```python
from build123d import *

# Parameters (mm, degrees)
F0_R     = 1.5875
F1_DEPTH = 1.5875
F2_R     = 0.79375
F5_DEPTH = 1.5885


with BuildPart() as f1:
    # F0 (on Top) → F1 (new body)
    with BuildSketch(Plane.XY):
        with BuildLine():
            Line((0, 52.563247), (0, 0))
            Line((0, 0), (98.425, 0))
            Line((98.425, 0), (98.425, 46.388994))
            Line((98.425, 46.388994), (14.2875, 46.388994))
            Line((14.2875, 46.388994), (14.2875, 98.425))
            Line((14.2875, 98.425), (31.75, 98.425))
            ThreePointArc((31.75, 98.425), (44.45, 111.125), (31.75, 123.825))
            Line((31.75, 123.825), (0, 123.825))
            Line((0, 123.825), (0, 92.250747))
            ThreePointArc((0, 92.250747), (2.80633, 91.088327), (3.96875, 88.281997))
            Line((3.96875, 88.281997), (3.96875, 56.531997))
            ThreePointArc((3.96875, 56.531997), (2.80633, 53.725667), (0, 52.563247))
        make_face()
        with BuildLine():
            Line((71.4375, 6.35), (39.6875, 6.35))
            ThreePointArc((39.6875, 6.35), (35.71875, 10.31875), (39.6875, 14.2875))
            Line((39.6875, 14.2875), (71.4375, 14.2875))
            ThreePointArc((71.4375, 14.2875), (75.40625, 10.31875), (71.4375, 6.35))
        make_face(mode=Mode.SUBTRACT)
        with BuildLine():
            Line((71.4375, 31.307744), (39.6875, 31.307744))
            ThreePointArc((39.6875, 31.307744), (35.71875, 35.276494), (39.6875, 39.245244))
            Line((39.6875, 39.245244), (71.4375, 39.245244))
            ThreePointArc((71.4375, 39.245244), (75.40625, 35.276494), (71.4375, 31.307744))
        make_face(mode=Mode.SUBTRACT)
        with Locations((31.75, 111.125)):
            Circle(F0_R, mode=Mode.SUBTRACT)
        with BuildLine():
            ThreePointArc((39.6875, 39.245244), (35.71875, 35.276494), (39.6875, 31.307744))
            Line((39.6875, 31.307744), (71.4375, 31.307744))
            ThreePointArc((71.4375, 31.307744), (75.40625, 35.276494), (71.4375, 39.245244))
            Line((71.4375, 39.245244), (39.6875, 39.245244))
        make_face()
        with BuildLine():
            ThreePointArc((39.6875, 14.2875), (35.71875, 10.31875), (39.6875, 6.35))
            Line((39.6875, 6.35), (71.4375, 6.35))
            ThreePointArc((71.4375, 6.35), (75.40625, 10.31875), (71.4375, 14.2875))
            Line((71.4375, 14.2875), (39.6875, 14.2875))
        make_face()
    extrude(amount=F1_DEPTH)

    # F2
    f2_edges = [f1.edges().sort_by_distance(p)[0] for p in [
        (14.2875, 98.425, 0.79375),
        (14.2875, 46.388994, 0.79375),
        (98.425, 46.388994, 0.79375),
        (98.425, 0, 0.79375),
    ]]
    fillet(f2_edges, radius=F2_R)

    # F3: F1 across plane


with BuildPart() as f1_1:
    add(f1.part)
    add(f1.part.mirror(Plane.YZ))

    # F4 (on face) → F5 (cut, through all)
    with BuildSketch(Plane.XY.offset(1.5875)):
        with BuildLine():
            ThreePointArc((-71.4375, 27.163247), (-75.40625, 23.194497), (-71.4375, 19.225747))
            Line((-71.4375, 19.225747), (-39.6875, 19.225747))
            ThreePointArc((-39.6875, 19.225747), (-35.71875, 23.194497), (-39.6875, 27.163247))
            Line((-39.6875, 27.163247), (-71.4375, 27.163247))
        make_face()
        with BuildLine():
            Line((71.4375, 39.245244), (39.6875, 39.245244))
            ThreePointArc((39.6875, 39.245244), (35.71875, 35.276494), (39.6875, 31.307744))
            Line((39.6875, 31.307744), (71.4375, 31.307744))
            ThreePointArc((71.4375, 31.307744), (75.40625, 35.276494), (71.4375, 39.245244))
        make_face()
        with BuildLine():
            ThreePointArc((39.6875, 14.2875), (35.71875, 10.31875), (39.6875, 6.35))
            Line((39.6875, 6.35), (71.4375, 6.35))
            ThreePointArc((71.4375, 6.35), (75.40625, 10.31875), (71.4375, 14.2875))
            Line((71.4375, 14.2875), (39.6875, 14.2875))
        make_face()
    extrude(amount=-F5_DEPTH, mode=Mode.SUBTRACT)


solid = f1_1.part
```
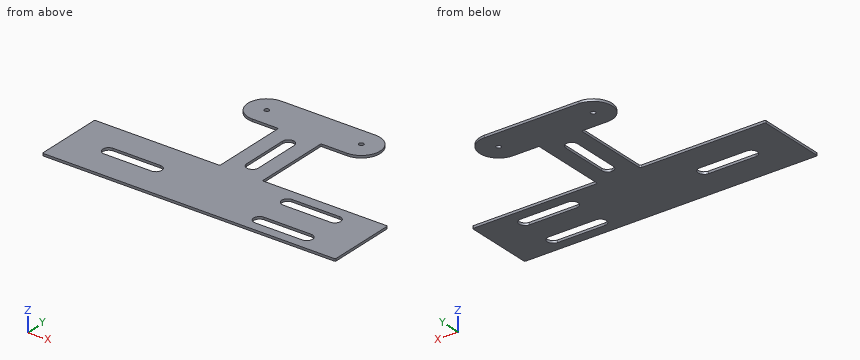
Model file for the job. Use its own axes, mm. Give positions to 0.01 mm unless a question says otherwise; leave off trailing zeros. Loops run counter-clockwise (first coordinate to the right, second up) from the corner with the lowest first, then second, coordinate; pieces in that order, holes last. Notation, with made-up numbers: (54.5, -28) -> (66.5, -28) arc R23 cw to (66.5, 4) -> close; hole circle Ø8 at (-27.5, 9.5). An arc over 180 degrees is marked (long way). Write each question's results on one line, items separated by ' | '.
(1) Cut at D-D on y = 95. List the corners of the cut face in (x, z).
Geometry results:
outline: (-14.29, 0) -> (14.29, 0) -> (14.29, 1.59) -> (-14.29, 1.59) -> close
(2) Cut at B-B on y = 24.5. List the corners of the cut face in (x, z) (1 decimal).
Geometry results:
outline: (-98.4, 0) -> (-75.2, 0) -> (-75.2, 1.6) -> (-98.4, 1.6) -> close; (-35.9, 0) -> (98.4, 0) -> (98.4, 1.6) -> (-35.9, 1.6) -> close
(3) Cut at A-A on y = 73.5. List the corners of the cut face in (x, z), and give its area (3 significant figures).
Geometry results:
outline: (-14.29, 0) -> (-3.97, 0) -> (-3.97, 1.59) -> (-14.29, 1.59) -> close; (3.97, 0) -> (14.29, 0) -> (14.29, 1.59) -> (3.97, 1.59) -> close | area: 32.8 mm²
(4) Cut at C-C on z = 1.05. Give the number of separate pieces and of enclosed holes in the cut face, and give its area (3 significant figures).
Geometry results:
separate pieces: 1 | enclosed holes: 6 | area: 11,500 mm²
(5) Probe line 1 along Y through (x, z) = (-31.75, 0.7) (1 decimal); line 2 along X through (y, z) = (60, 1.2); line 3 along Y through (x, z) = (-33, 1.4). List the from-to ranges inside material, lowest first.
Geometry results:
line 1: y = 0 to 46.4, 98.4 to 109.5, 112.7 to 123.8 | line 2: x = -14.29 to -3.97, 3.97 to 14.29 | line 3: y = 0 to 46.39, 98.49 to 110.15, 112.1 to 123.76
(6) Flat gauge pins, fed straight in: pin 1 Ø2.5 at (x, y) = (31.75, 111.125) entering from +Z; pin 2 Ø0.8 at (y, z) = (60.5, 0.5) entering from -X; pin 3 Ø0.5 at (x, z) = (56, 0.5) entering from +Y. Where does each tip first touch, or does it go through?
Geometry results:
pin 1: passes through | pin 2: stops at x = -14.29 | pin 3: stops at y = 46.39
